Input: part model. Units: mm. Frame: model coordinates. Face numbers are marked on the shaded views. A direction names the side the tool comes from. Round coordinates to 2 decimals unless told otherwise and drop trailing zeros. Write each loop counter-clockwise with the first axis right and the second up, starting at its lowest first coordinate (ties: lowest second). Pieces come first, ordered by that corner, then holes. Notation, with made-up numbers: M 65,63.25 L 96,63.25 A25 ccw 96,93.25 Z; hole C 22.5,87 d11. An arc over 180 degrees is marked long. Answer as CSV lines item,"result". Start each with the question number.
```python
from build123d import *

# Parameters (mm, degrees)
SKETCH_W      = 60
SKETCH_H      = 40
PAD_DEPTH     = 2
SKETCH001_W   = 60
SKETCH001_H   = 40
SKETCH001_W_2 = 44
SKETCH001_H_2 = 24
PAD001_DEPTH  = 10
SKETCH002_W   = 58
SKETCH002_H   = 38
SKETCH002_W_2 = 54.8
SKETCH002_H_2 = 34.8
SKETCH002_R   = 1.4
POCKET_DEPTH  = 6


with BuildPart() as part:
    # Sketch → Pad (new body)
    with BuildSketch(Plane.XY):
        Rectangle(SKETCH_W, SKETCH_H)
    extrude(amount=PAD_DEPTH)

    # Sketch001 → Pad001 (join)
    with BuildSketch(Plane.XY):
        Rectangle(SKETCH001_W, SKETCH001_H)
        Rectangle(SKETCH001_W_2, SKETCH001_H_2, mode=Mode.SUBTRACT)
    extrude(amount=PAD001_DEPTH)

    # Sketch002 (on Face10 of Pad001) → Pocket (cut)
    with BuildSketch(Plane.XY.offset(10)):
        Rectangle(SKETCH002_W, SKETCH002_H)
        Rectangle(SKETCH002_W_2, SKETCH002_H_2, mode=Mode.SUBTRACT)
        with Locations((0, 14.6)):
            Circle(SKETCH002_R)
        with Locations((24.6, 0)):
            Circle(SKETCH002_R)
        with Locations((0, -14.6)):
            Circle(SKETCH002_R)
        with Locations((-24.6, 0)):
            Circle(SKETCH002_R)
    extrude(amount=-POCKET_DEPTH, mode=Mode.SUBTRACT)


solid = part.part
```
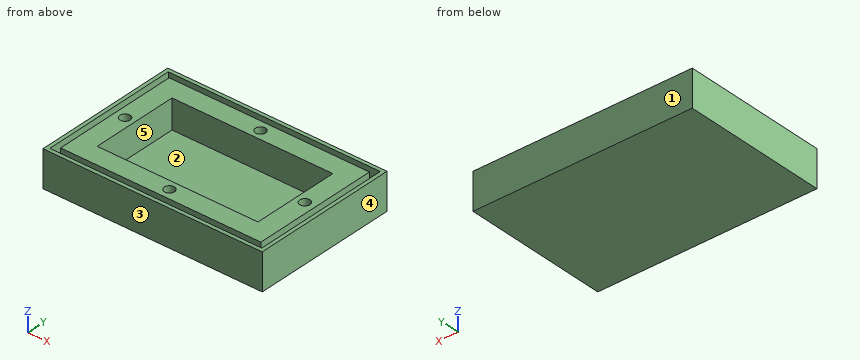
Item 1: Cut plane C-C, the plane x = -24.6. Return loops of the section in (y, z), plus the area to 3 significant figures.
Item 2: Pin query (flat end, axial travel): pin 1 Ø12 at (x, y) = (-10.5, 14.5) entering from -Z; pin 2 Ø2.5 at (x, y) = (24.6, 0) entering from +Z; pin 3 Ø8 at (x, y) = (-12.5, 3) entering from +Z. Return the tip coordinate at first contact, or that it passes through.
Item 3: Access query for the marked faces 4 and 5. Directions: +Z, -Z, +X, -X, +Y, -Y. A direction counts if a zero-diameter tool reaches every point of the face in a straight line with its end or side. Return the directions, or none.
Item 4: Draft query along Y for the marked faces 1, 2 and 3. Return one class per face: +Y half, -Y half, draft (parallel to the pull), parting line (faces both ways), or undercut.
Item 5: Cut plane A-A, the plane z = 8.75. Return loops of the section in (x, y), plus the area to 3 significant figures.
Item 6: Cut plane B-B, the plane y = 14.6. Return loops of the section in (x, z).
Item 7: Line query: line 1 (Y direction, x = 3.5, z = 7.25); line 2 (Y direction, x = 0, z = 7.5); line 3 (Y direction, x = 24.6, z = 6.2). Output: solid intervals per line, ascending. Write a range as [from, to].
Item 8: Cut plane D-D, the plane z = 3. Return loops of the section in (x, y).
Results list:
1,outline,"M -20,0 L 20,0 L 20,10 L 19,10 L 19,4 L 17.4,4 L 17.4,10 L 1.4,10 L 1.4,4 L -1.4,4 L -1.4,10 L -17.4,10 L -17.4,4 L -19,4 L -19,10 L -20,10 Z"
1,area,"364 mm²"
2,pin 1,"z = 0"
2,pin 2,"z = 4"
2,pin 3,"z = 2"
3,face 4,"+Z, -Z, +X, +Y, -Y"
3,face 5,"+Z"
4,face 1,"+Y half"
4,face 2,"undercut"
4,face 3,"-Y half"
5,outline,"M -30,-20 L 30,-20 L 30,20 L -30,20 Z; M -27.4,-17.4 L 27.4,-17.4 L 27.4,17.4 L -27.4,17.4 Z; hole M -29,-19 L 29,-19 L 29,19 L -29,19 Z; hole C -24.6,0 d2.8; hole M -22,-12 L 22,-12 L 22,12 L -22,12 Z; hole C 0,-14.6 d2.8; hole C 0,14.6 d2.8; hole C 24.6,0 d2.8"
5,area,"1,020 mm²"
6,outline,"M -30,0 L 30,0 L 30,10 L 29,10 L 29,4 L 27.4,4 L 27.4,10 L 1.4,10 L 1.4,4 L -1.4,4 L -1.4,10 L -27.4,10 L -27.4,4 L -29,4 L -29,10 L -30,10 Z"
7,line 1,"[-20, -19], [-17.4, -12], [12, 17.4], [19, 20]"
7,line 2,"[-20, -19], [-17.4, -16], [-13.2, -12], [12, 13.2], [16, 17.4], [19, 20]"
7,line 3,"[-20, -19], [-17.4, -1.4], [1.4, 17.4], [19, 20]"
8,outline,"M -30,-20 L 30,-20 L 30,20 L -30,20 Z; hole M -22,-12 L 22,-12 L 22,12 L -22,12 Z"
